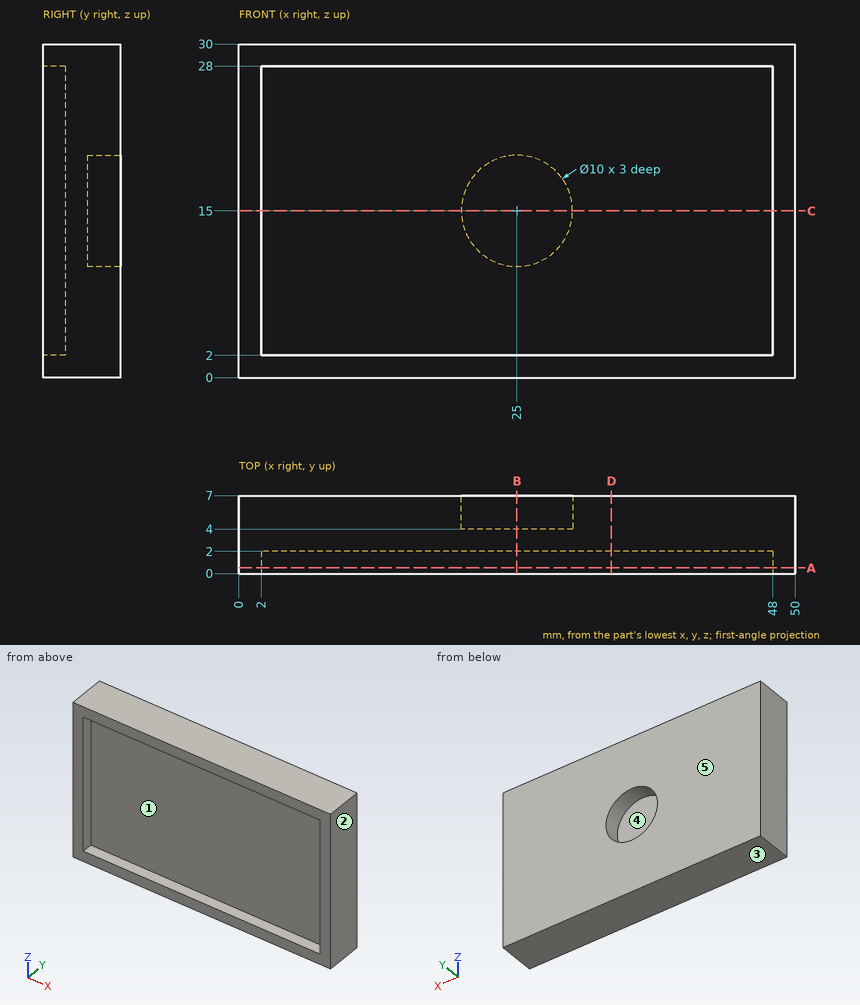
For this review, use the dimensioned drawing (mm, ordinates from the lowest corner) and the shaded views. A direction names the side the tool comes from. Round coordinates to 2 decimals unless told otherwise and drop trailing zeros. Write each loop counter-clockwise with the first axis right and the second up, starting at its lowest first coordinate (ties: lowest second). Pieces come first, ordered by that corner, then holes. Notation, with made-up numbers: (15, 86.5) - (28, 86.5) arc R23 ccw to (28, 99.5) - close; hole circle Ø8 at (-3, -13.5). An arc over 180 degrees is marked (long way). One line per item, written item: value. Start each with the question number.
1. Consider section B-B on x = 25. Write out the cut boundary in (y, z), and give its area (3 significant figures).
2. Consider section A-A on y = 0.5. Write out the cut boundary in (x, z), and give its area (3 significant figures).
3. Consider section C-C on z = 15. Write out the cut boundary in (x, y).
4. The part is to be moulded in two halves that separate along Z. For the marked faces 3, 4 and 5, say which applies: released by +Z, released by -Z, zero draft, split by the parting line, or undercut.
5. Clearance check with flat-ended pins moving along their axes: P1, Ø13, axis at x = 36, z = 18.5, coming from the -Y side; P2, Ø5, axis at x = 24.5, z = 14, coming from the +Y side. State where each tip first meets the part, or that it passes through.
6. Consider section D-D on x = 33.5. Write out the cut boundary in (y, z), and give its area (3 significant figures).
7. Machinability: for the marked faces 1 and 2, which of the approach directions +Z, -Z, +X, -X, +Y, -Y give a long, thin tool a straight path to every point of the face, cutting with its end or side? Answer none if there is none.
8. To check wall thickness, follow L1, parallel to X at y = 1.5, z = 25.5; L2, parallel to Z at x = 25, y = 5.35; L3, parallel to Z at x = 17, y = 0.5. State the ranges of each line that lie inside material, in increasing order. Write a range as from..to.
Checks:
1. outline: (0, 0) - (7, 0) - (7, 10) - (4, 10) - (4, 20) - (7, 20) - (7, 30) - (0, 30) - (0, 28) - (2, 28) - (2, 2) - (0, 2) - close
1. area: 128 mm^2
2. outline: (0, 0) - (50, 0) - (50, 30) - (0, 30) - close; hole (2, 2) - (48, 2) - (48, 28) - (2, 28) - close
2. area: 304 mm^2
3. outline: (0, 0) - (2, 0) - (2, 2) - (48, 2) - (48, 0) - (50, 0) - (50, 7) - (30, 7) - (30, 4) - (20, 4) - (20, 7) - (0, 7) - close
4. face 3: released by -Z
4. face 4: undercut
4. face 5: zero draft
5. P1: stops at y = 2
5. P2: stops at y = 4
6. outline: (0, 0) - (7, 0) - (7, 30) - (0, 30) - (0, 28) - (2, 28) - (2, 2) - (0, 2) - close
6. area: 158 mm^2
7. face 1: -Y
7. face 2: +Z, -Z, +X, +Y, -Y
8. L1: x = 0..2, 48..50
8. L2: z = 0..10, 20..30
8. L3: z = 0..2, 28..30
